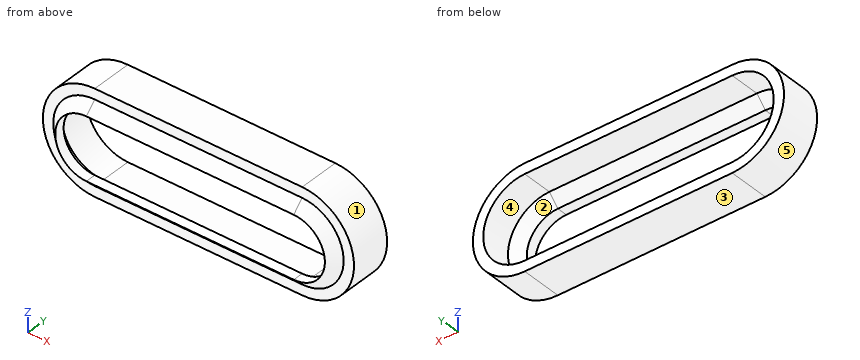
from build123d import *

# Parameters (mm, degrees)
BOSS_EXTRUDE1_DEPTH      = 10
BOSS_EXTRUDE2_DEPTH      = 2.54
BOSS_EXTRUDE2_DEPTH_BACK = 2.54
CHAMFER1_SIZE            = 2.54


with BuildPart() as part:
    # Sketch1 → Boss-Extrude1 (new body)
    with BuildSketch(Plane(origin=(0, 0, 0), x_dir=(1, 0, 0), z_dir=(0, 1, 0))):
        with BuildLine():
            Line((-25.4, -12.7), (25.4, -12.7))
            ThreePointArc((25.4, -12.7), (38.1, 0), (25.4, 12.7))
            Line((25.4, 12.7), (-25.4, 12.7))
            ThreePointArc((-25.4, 12.7), (-38.1, 0), (-25.4, -12.7))
        make_face()
        with BuildLine():
            Line((-25.4, -10.16), (25.4, -10.16))
            ThreePointArc((25.4, -10.16), (35.56, 0), (25.4, 10.16))
            Line((25.4, 10.16), (-25.4, 10.16))
            ThreePointArc((-25.4, 10.16), (-35.56, 0), (-25.4, -10.16))
        make_face(mode=Mode.SUBTRACT)
    extrude(amount=BOSS_EXTRUDE1_DEPTH)

    # Sketch3 → Boss-Extrude2 (add, two sides: drawn at the far end of the back side and taken through both)
    with BuildSketch(Plane.XZ.offset(-BOSS_EXTRUDE2_DEPTH_BACK)):
        with BuildLine():
            Line((25.4, 10.16), (-25.4, 10.16))
            ThreePointArc((-25.4, 10.16), (-35.56, 0), (-25.4, -10.16))
            Line((-25.4, -10.16), (25.4, -10.16))
            ThreePointArc((25.4, -10.16), (35.56, 0), (25.4, 10.16))
        make_face()
        with BuildLine():
            Line((-25.4, -7.62), (25.4, -7.62))
            ThreePointArc((25.4, -7.62), (33.02, 0), (25.4, 7.62))
            Line((25.4, 7.62), (-25.4, 7.62))
            ThreePointArc((-25.4, 7.62), (-33.02, 0), (-25.4, -7.62))
        make_face(mode=Mode.SUBTRACT)
    extrude(amount=BOSS_EXTRUDE2_DEPTH + BOSS_EXTRUDE2_DEPTH_BACK)

    # Chamfer1
    chamfer1_edges = [part.edges().sort_by_distance(p)[0] for p in [
        (35.56, -2.54, 0),
        (0, -2.54, 10.16),
        (0, -2.54, -10.16),
        (-35.56, -2.54, 0),
        (0, 2.54, 7.62),
        (-33.02, 2.54, 0),
        (33.02, 2.54, 0),
        (0, 2.54, -7.62),
    ]]
    chamfer(chamfer1_edges, length=CHAMFER1_SIZE - 0.0001)  # a hair under: the kernel refuses the full size


solid = part.part
Geometry check sheet. Reference: the model listing, model coordinates, mm. Face numbers are marked on the shaded views. A direction names the side the tool comes from. Coordinates: 2 decimals unless noted, no trailing zeros. Order: outer loops, then holes, each group sorted by start corner. A loop starts at its lowest first (then second) coordinate and runs counter-clockwise, first axis right, second up. Notation, with made-up numbers: (40, 75.25) -> (62, 75.25) arc R11 ccw to (62, 79.25) -> close; hole circle Ø6 at (5.5, 45.25). An arc over 180 degrees is marked (long way). Use a Markdown table: item, result. Add a question column.
1. Cross-section at C-C (y = 8.25). Enter the section's corners in (x, z), and give its area (3 significant figures).
2. Set-up check for the marked faces 4 and 5: record each of +Z, -Z, +X, -X, +Y, -Y from which the full face is reachable in a straight line by a thin tool's end or side.
3. Material ranges on L1, parallel to Z at x = 8.5, y = 5; L2, parallel to Z at x = -14, y = -0.75; L3, parallel to X at y = -1.25, z = 0.25, recorded low to high.
4. Mould release check, pull along Z, two halves, no side actions. Record for the marked faces 1, 2 and 3: pulls with the +Z half, pulls with the -Z half, needs draft (parallel to the pull), parting line crosses it, or undercut.
5. Go/stop test with flat-tipped pins: pin 1 Ø3 at (x, y) = (6, -1) entering from +Z; pin 2 Ø3 at (y, z) = (7.5, -5.5) entering from -X; pin 3 Ø10 at (x, z) = (-9, -1) entering from -Y; pin 4 Ø2 at (x, y) = (-7.5, -1.5) entering from -Z. Record where each tip stops, or that it passes through.
Filled sheet:
| question | item | result |
|---|---|---|
| 1 | outline | (-25.4, -12.7) -> (25.4, -12.7) arc R12.7 ccw to (25.4, 12.7) -> (-25.4, 12.7) arc R12.7 ccw to start; hole (-25.4, -10.16) -> (25.4, -10.16) arc R10.16 ccw to (25.4, 10.16) -> (-25.4, 10.16) arc R10.16 ccw to start |
| 1 | area | 440 mm2 |
| 2 | face 4 | +Y |
| 2 | face 5 | -X, +Y, -Y |
| 3 | L1 | -12.7 to -10.16, 10.16 to 12.7 |
| 3 | L2 | -9.41 to -7.62, 7.62 to 9.41 |
| 3 | L3 | -34.31 to -33.02, 33.02 to 34.31 |
| 4 | face 1 | parting line crosses it |
| 4 | face 2 | undercut |
| 4 | face 3 | pulls with the -Z half |
| 5 | pin 1 | z = 12.7 |
| 5 | pin 2 | x = -37.45 |
| 5 | pin 3 | through |
| 5 | pin 4 | z = -9.66 |
